Read the model definition and answer for the solid it produces. Units are mm, in the model's axes. A direction names the side the tool comes from. Give positions to 0.01 mm unless a question says otherwise; leave off trailing zeros. Loops run counter-clockwise (first coordinate to the right, second up) from the corner with the lowest first, then second, coordinate; pieces in that order, holes last.
(1) Determine the mould class of faces 4 (the face through (-0.2, -11.5, 0.5)), 5 (the face through (0.2, -17.5, 2)), 6 (the face through (15.5, 0, 2)) for opening direction X: pulls with the +X half, pulls with the -X half, needs draft (parallel to the pull), parting line crosses it, or undercut.
(2) Find section B-B, the plane x = 6. Write down the section's boundary in (y, z).
(3) Find section A-A, the plane y = -10.5. Write down the section's boundary in (x, z).
(4) Straight lines are drawn through the part: probe 1 along X at (y, z) = (3.5, 0.65); probe 2 along X at (y, z) = (6, 1.9); probe 3 along Y at (x, z) = (-0.5, 2.4). For each, find the intervals that lie inside material, in ascending order.
(5) Find section C-C, the plane y = 12. Write down the section's boundary in (x, z), then the cut area to 3 significant figures.
(6) Which of the six approach directions +Z, -Z, +X, -X, +Y, -Y give full straight-line access (tool end or side, diameter ignored) to faces 1 (the face through (-11.5, -0.2, 0.5)), 2 (the face through (0, -13, 4)), 3 (the face through (12.5, 0, 3))?
(7) Find section D-D, the plane z = 3. Write down the section's boundary in (x, y).
(8) Each of these flat-tipped pins is pushed along its axis until it touches: P1, Ø1, axis at x = 9, z = 2, coming from the +Y side; P2, Ø7.5, axis at x = 4.5, y = -4.5, coming from the +Z side; P3, Ø10, axis at x = 9.5, y = 8, coming from the +Z side; P4, Ø1.1, axis at x = 1, z = 0.5, coming from the -Y side. Where does it stop, or does it pass through?
```python
from build123d import *

# Parameters (mm, degrees)
SKETCH3_W           = 31
SKETCH3_H           = 31
BOSS_EXTRUDE2_DEPTH = 4
SKETCH4_W           = 25
SKETCH4_H           = 25
CUT_EXTRUDE1_DEPTH  = 3
SKETCH5_W           = 23
SKETCH5_H           = 23
CUT_EXTRUDE2_DEPTH  = 5


with BuildPart() as part:
    # Sketch3 → Boss-Extrude2 (new body)
    with BuildSketch(Plane.XY):
        Rectangle(SKETCH3_W, SKETCH3_H)
    extrude(amount=BOSS_EXTRUDE2_DEPTH)

    # Sketch4 → Cut-Extrude1 (cut)
    with BuildSketch(Plane.XY.offset(4)):
        Rectangle(SKETCH4_W, SKETCH4_H)
    extrude(amount=-CUT_EXTRUDE1_DEPTH, mode=Mode.SUBTRACT)

    # Sketch5 → Cut-Extrude2 (cut)
    with BuildSketch(Plane.XY.offset(1)):
        Rectangle(SKETCH5_W, SKETCH5_H)
    extrude(amount=-CUT_EXTRUDE2_DEPTH, mode=Mode.SUBTRACT)

    # Sweep1: sweep along a curve in space
    with BuildLine() as sweep1_path:
        Line((-15.5, -15.5, 4), (15.5, -15.5, 4))
    # Sketch6 → Sweep1 (sweep)
    with BuildSketch(Plane.ZY.offset(15.5)):
        Polygon((4, -15.5), (4, -19.5), (0, -15.5), align=None)
    sweep(path=sweep1_path.line)

    # Sweep2: sweep along a curve in space
    with BuildLine() as sweep2_path:
        Line((15.5, 15.5, 0), (-15.5, 15.5, 0))
    # Sketch8 → Sweep2 (sweep)
    with BuildSketch(Plane.ZY.offset(15.5)):
        Polygon((0, 15.5), (4, 19.43634716), (4, 15.5), align=None)
    sweep(path=sweep2_path.line)


solid = part.part
```
Entries:
1. face 4: undercut
1. face 5: needs draft
1. face 6: pulls with the +X half
2. outline: (-19.5, 4) - (-15.5, 0) - (-11.5, 0) - (-11.5, 1) - (-12.5, 1) - (-12.5, 4) - close; (11.5, 0) - (15.5, 0) - (19.44, 4) - (12.5, 4) - (12.5, 1) - (11.5, 1) - close
3. outline: (-15.5, 0) - (-11.5, 0) - (-11.5, 1) - (-12.5, 1) - (-12.5, 4) - (-15.5, 4) - close; (11.5, 0) - (15.5, 0) - (15.5, 4) - (12.5, 4) - (12.5, 1) - (11.5, 1) - close
4. probe 1: x = -15.5 to -11.5, 11.5 to 15.5
4. probe 2: x = -15.5 to -12.5, 12.5 to 15.5
4. probe 3: y = -17.9 to -12.5, 12.5 to 17.86
5. outline: (-15.5, 0) - (15.5, 0) - (15.5, 4) - (12.5, 4) - (12.5, 1) - (-12.5, 1) - (-12.5, 4) - (-15.5, 4) - close
5. area: 49.0 mm2
6. face 1: +Z, -Z
6. face 2: +Z, +X, -X, +Y, -Y
6. face 3: +Z
7. outline: (-15.5, -18.5) - (15.5, -18.5) - (15.5, 18.45) - (-15.5, 18.45) - close; hole (-12.5, -12.5) - (12.5, -12.5) - (12.5, 12.5) - (-12.5, 12.5) - close
8. P1: stops at y = 17.96
8. P2: passes through
8. P3: stops at z = 4
8. P4: stops at y = -16.55
